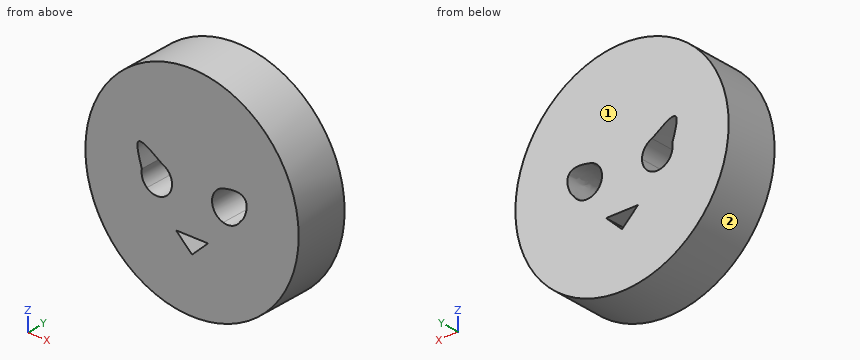
from build123d import *

# Parameters (mm, degrees)
F0_R     = 50.8
F1_DEPTH = 25.4


with BuildPart() as f1:
    # F0 (on Front) → F1 (new body)
    with BuildSketch(Plane.XZ):
        Circle(F0_R)
        Polygon((0, -25.4), (-7.6217073622, -18.1220550468), (7.6217073622, -18.1220550468), align=None, mode=Mode.SUBTRACT)
        with BuildLine():
            ThreePointArc((-14.2554945443, 6.803100084), (-10.8238557625, 4.1430589359), (-9.525, 0))
            ThreePointArc((-9.525, 0), (-13.7319278898, -6.5850065377), (-21.475243217, -5.5354251383))
            ThreePointArc((-21.475243217, -5.5354251383), (-23.6314387915, -2.3985970176), (-23.9033384682, 1.3981042586))
            add(Edge.make_bspline(
                [(-14.2554945443, 6.803100084), (-19.0561525649, 10.0658788244), (-27.9600989694, 16.1266078405), (-25.6616575186, 6.7049880874), (-23.9033384682, 1.3981042586)],
                knots=[0, 0, 0, 0, 0.4524785293, 0.8394989496, 0.8394989496, 0.8394989496, 0.8394989496], degree=3))
        make_face(mode=Mode.SUBTRACT)
        with BuildLine():
            ThreePointArc((14.839976255, -6.9924324336), (9.525236299, 0.0585632534), (14.9530797492, 7.0228662664))
            add(Edge.make_bspline(
                [(14.9530797492, 7.0228662664), (27.0596550391, 10.175950689), (26.5589054798, 1.2219851028), (24.153074938, -2.7644417195), (23.0182577745, -3.7117372195)],
                knots=[0, 0, 0, 0, 0.4992357934, 0.7063104799, 0.7063104799, 0.7063104799, 0.7063104799], degree=3))
            ThreePointArc((23.0182577745, -3.7117372195), (19.4840381744, -6.7354201163), (14.839976255, -6.9924324336))
        make_face(mode=Mode.SUBTRACT)
    extrude(amount=F1_DEPTH)


solid = f1.part
The listing builds one solid part. Answer for the finished solid, in the listing's coordinates (mm). Face numbers are marked on the shaded views. Round coordinates to 2 decimals unless told otherwise and drop trailing zeros. Write each loop counter-clockwise with the first axis right and the second up, starting at its lowest first coordinate (ties: lowest second). Pieces come first, ordered by that corner, then holes. Notation, with made-up numbers: (-5, 79.25) - (43, 79.25) arc R8 cw to (43, 87.25) - close; hole circle Ø3 at (-24, 28). An arc over 180 degrees is marked (long way). Use one line per item in the form item = value. Start each with the question number.
Item 1: A cutting plane is placed at C-C (x = 40). Write down the section's boundary in (y, z), plus the area to 3 significant figures.
Item 2: Flat-ended cylindrical pins translate along their axes: pin 1 Ø1.5 at (x, y) = (-21, -15.5) entering from -Z; pin 2 Ø6 at (x, y) = (-19, -14) entering from -Z; pin 3 Ø12 at (x, y) = (-1.5, -11) entering from -Z. Find the tip coordinate at first contact, or state that the pin passes through.
Item 3: A cutting plane is placed at A-A (y = -18.25). Give the number of separate pieces and of enclosed holes in the cut face, plus the area to 3 significant figures.
Item 4: Find the intervals of material crossed by line 1 (Z direction, x = 0, y = -24); line 2 (X direction, y = -3, z = 6.5); line 3 (X direction, y = -11.5, z = 1), in increasing order. Write a range as [from, to].
Item 5: Determine the mould class of the marked faces 1 and 2 for opening direction X: +X half, -X half, draft (parallel to the pull), parting line (faces both ways), or undercut.
Item 6: A cutting plane is placed at B-B (z = 31.5). Write down the section's boundary in (x, y), plus the area to 3 significant figures.
The answers:
q1.outline = (-25.4, -31.32) - (0, -31.32) - (0, 31.32) - (-25.4, 31.32) - close
q1.area = 1,590 mm^2
q2.pin_1 = -46.59
q2.pin_2 = -48.21
q2.pin_3 = -50.8
q3.separate_pieces = 1
q3.enclosed_holes = 3
q3.area = 7,640 mm^2
q4.line_1 = [-50.8, -25.4], [-18.12, 50.8]
q4.line_2 = [-50.38, -25.42], [-13.55, 13.55], [24.89, 50.38]
q4.line_3 = [-50.79, -23.97], [-9.59, 9.59], [25.7, 50.79]
q5.face_1 = draft
q5.face_2 = parting line
q6.outline = (-39.85, -25.4) - (39.85, -25.4) - (39.85, 0) - (-39.85, 0) - close
q6.area = 2,020 mm^2
